Autodesk Inventor part; units mm, degrees
ref_plane "YZ Plane" through (0, 0, 0) normal (1, 0, 0) x (0, 1, 0)
ref_plane "XZ Plane" through (0, 0, 0) normal (0, 1, 0) x (-1, 0, 0)
ref_plane "XY Plane" through (0, 0, 0) normal (0, 0, 1) x (1, 0, 0)
sketch "Sketch1" plane through (0, 0, 0) normal (0, 0, 1) x (1, 0, 0)
  line L0 (0, 0) -> (-156, 0)
  line L1 (0, 0) -> (0, 14.5)
  line L2 (0, 14.5) -> (-3, 17.5)
  line L3 (-3, 17.5) -> (-142, 17.5)
  line L4 (-142, 17.5) -> (-142, 25)
  line L5 (-142, 25) -> (-155, 25)
  line L6 (-155, 25) -> (-156, 24)
  line L7 (-156, 24) -> (-156, 0)
  dimension "d0" = 35
  dimension "d1" = 3
  dimension "d2" = 45
  dimension "d4" = 14
  dimension "d5" = 156
  dimension "d6" = 50
  dimension "d7" = 45
  dimension "d8" = 1
revolve "Revolution1" add sketch "Sketch1" angle 360 about axis through (0, 0, 0) along (-1, 0, 0)
sketch "Sketch2" plane through (-156, 0, 0) normal (-1, 0, 0) x (0, 0, 1)
  circle A0 centre (0, 0) radius 24
  point P0 (0, 0)
hole "Hole1" at (-156, 0, 0) direction (1, 0, 0) diameter 8 depth 80 tip angle 118
sketch "Sketch3" plane through (0, 0, 0) normal (0, 0, 1) x (1, 0, 0)
  line L0 (-156, -24) -> (-156, 24)
  line L1 (-156, 7) -> (-155, 6)
  line L2 (-155, 6) -> (-140, 6)
  line L3 (-140, 6) -> (-140, 4)
  line L4 (-76, 4) -> (-156, 4)
  line L5 (-156, 0) -> (-73.5966, 0)
  line L6 (-73.5966, 0) -> (-76, -4)
  point P0 (0, 0)
  dimension "d17" = 1
  dimension "d18" = 6
  dimension "d19" = 16
  dimension "d20" = 45
revolve "Revolution2" cut sketch "Sketch3" angle 360 about axis through (-156, 0, 0) along (1, 0, 0)
sketch "Sketch4" plane through (0, 0, 0) normal (0, 0, 1) x (1, 0, 0)
  line L0 (-142, 17.5) -> (-3, 17.5)
  line L1 (-12, 17.5) -> (-12, 9.5)
  line L2 (-12, 9.5) -> (-8, 9.5)
  line L3 (-8, 9.5) -> (-8, 17.5)
  line L4 (0, -14.5) -> (0, 14.5)
  point P0 (0, 0)
  dimension "d22" = 4
  dimension "d23" = 12
  dimension "d24" = 8
extrude "Extrusion1" cut sketch "Sketch4" along normal through all both and the other way through all
sketch "Sketch5" plane through (0, 0, 0) normal (0, 0, 1) x (1, 0, 0)
  line L0 (-76, 4) -> (-140, 4)
  line L1 (-81, 4) -> (-81, 17.5)
  line L2 (-142, 17.5) -> (-3, 17.5)
  line L3 (-77, 17.5) -> (-77, 4)
  line L4 (-156, -24) -> (-156, 24)
  line L5 (-76, -4) -> (-140, -4)
  line L6 (-81, 4) -> (-81, -4)
  line L7 (-76, 4) -> (-140, 4)
  line L8 (-77, 4) -> (-77, -4)
  line L9 (-81, 0) -> (-77, 0)
  line L10 (-77, 13.5) -> (-81, 13.5)
  point P0 (0, 0)
  dimension "d27" = 4
  dimension "d28" = 75
  dimension "d33" = 4
revolve "Revolution3" cut sketch "Sketch5" angle 360 about axis through (-81, 4, 0) along (0, 1, 0) contours L8 L9 L6 L0 | L0 L1 L10 L3 | L10 L1 L2 L3
sketch "Sketch6" plane through (0, 0, 0) normal (0, 0, 1) x (1, 0, 0)
  line L0 (-142, 17.5) -> (-3, 17.5)
  line L1 (-106, 17.5) -> (-106, 13.5)
  line L2 (-106, 13.5) -> (-81, 13.5)
  line L3 (-81, 13.5) -> (-56, 13.5)
  line L4 (-56, 13.5) -> (-56, 17.5)
  line L5 (-106, 17.5) -> (-56, 17.5)
  line L6 (-142, 17.5) -> (-3, 17.5)
  line L7 (-77, 4) -> (-81, 0)
  line L8 (-81, 17.5) -> (-81, 0)
  point P0 (0, 0)
  dimension "d30" = 50
  dimension "d31" = 4
revolve "Revolution4" cut sketch "Sketch6" angle 360 about axis through (-142, 17.5, 0) along (1, 0, 0)
properties part number "Ось" material "Steel, Cast"
Here's how the part is built. I have some questions about the finished solid (model axes, mm). A direction names the side the tool comes from. Round coordinates to 2 decimals unless told otherwise and drop trailing zeros. Order: outer loops, then holes, each group sorted by start corner. A loop starts at its lowest first (then second) coordinate and runs counter-clockwise, first axis right, second up. Notation, with made-up numbers: M -35,16.25 L -5,16.25 A14 ccw -5,24.25 Z; hole C 4,10.25 d3. An arc over 180 degrees is marked long. Answer in a Markdown table with one row per item.
Item 1: If I drill on L1, parallel to Y at x = -98, z = 0; L2, parallel to Z at x = -93.5, y = 0, over which ranges is the centre line in solid material (lowest first)? Write a range as from..to.
A:
| item | result |
|---|---|
| L1 | y = -17.5..-4, 4..13.5 |
| L2 | z = -17.5..-4, 4..17.5 |
Item 2: Imagine slicing it at A-A, the plane x = -113.5. Write out the boundary of the cut face in (y, z).
A:
| item | result |
|---|---|
| outline | C 0,0 d35; hole C 0,0 d8 |
Item 3: I'm going to push flat-ended pins straight in: pin 1 (1.5 mm diameter, centred on x = -71, z = -0.5, fed in from -Y); pin 2 (4.5 mm diameter, centred on x = -10, z = -6, fed in from +Y); pin 3 (13 mm diameter, centred on x = -81, z = 0, fed in from +Y); pin 4 (4.5 mm diameter, centred on y = 15, z = -0.5, fed in from +X). Where does each tip first touch, or does it pass through?
A:
| item | result |
|---|---|
| pin 1 | stops at y = -17.5 |
| pin 2 | stops at y = 16.78 |
| pin 3 | stops at y = 17.04 |
| pin 4 | stops at x = 0 |
Item 4: Imagine slicing it at B-B, the plane x = -38.5. Write out the boundary of the cut face in (y, z).
A:
| item | result |
|---|---|
| outline | C 0,0 d35 |
Item 5: For faces 1 (the face through (-10, 9.5, 0)), 2 (the face through (-140, -1.42, -3.92)), 3 (the face through (-93.6, 13.5, 0.1)), 4 (the face through (-73.473, -17.483, -0.769)), which set-ups out of +Z, -Z, +X, -X, +Y, -Y let a thin tool reach every point of the face, with its end or its side?
A:
| item | result |
|---|---|
| face 1 | +Z, -Z, +Y |
| face 2 | -X |
| face 3 | +Y |
| face 4 | +X |
Item 6: Imagine slicing it at C-C, the plane x = -86.5. Write out the boundary of the cut face in (y, z), and give its area (3 significant figures).
A:
| item | result |
|---|---|
| outline | M 17.04,-3.97 A4 cw 17.04,3.97 A17.5 ccw long Z; hole C 0,0 d8 |
| area | 888 mm2 |
Item 7: Thinking about a two-plate mould opening in Z: for faces 5 (the face through (-106, 16, 0)), 6 (the face through (-0.19, -3.18, 14.34)), 7 (the face through (-12, 13, 0)), 8 (the face through (-107.552, -3.373, 2.15)), which applies, +Z half, -Z half, draft (parallel to the pull), parting line (faces both ways), or undercut?
A:
| item | result |
|---|---|
| face 5 | undercut |
| face 6 | parting line |
| face 7 | draft |
| face 8 | undercut |
